from build123d import *

# Parameters (mm, degrees)
BOSS_EXTRUDE1_DEPTH = 10
SHELL1_START        = 1
SHELL1_DEPTH        = 9
CUT_EXTRUDE1_REACH  = 40.243
SKETCH2_W           = 4
SKETCH2_H           = 9


# Read off the part's stored shape, not the designer's step: Shell1
with BuildPart() as part:
    # Sketch1 → Boss-Extrude1 (new body)
    with BuildSketch(Plane.XY):
        with BuildLine():
            Line((-17.310520711, -21.823889376), (-3.597740248, -21.843555797))
            Line((-3.597740248, -21.843555797), (2.757908107, -14.842465178))
            ThreePointArc((2.757908107, -14.842465178), (-10.455115829, 18.525441507), (-23.668139764, -14.842465178))
            Line((-23.668139764, -14.842465178), (-17.310520711, -21.823889376))
        make_face()
    extrude(amount=BOSS_EXTRUDE1_DEPTH)

    # Shell1 outline → Shell1 (cut)
    with BuildSketch(Plane.XY.offset(SHELL1_START)):
        with BuildLine():
            Line((-4.039953619, -20.84292056), (2.044621953, -14.140431281))
            ThreePointArc((2.044621953, -14.140431281), (-10.45473176, 17.525441503), (-22.955414629, -14.139906596))
            Line((-22.955414629, -14.139906596), (-16.868083072, -20.824522877))
            Line((-16.868083072, -20.824522877), (-4.039953619, -20.84292056))
        make_face()
    extrude(amount=SHELL1_DEPTH, mode=Mode.SUBTRACT)

    # Sketch2 → Cut-Extrude1 (cut, up to next)
    with BuildSketch(Plane.XY.offset(10), mode=Mode.PRIVATE) as cut_extrude1_sk1:
        with Locations((-10.090473375, -2.029514736)):
            Rectangle(SKETCH2_W, SKETCH2_H)
    cut_extrude1_tool1 = extrude(cut_extrude1_sk1.sketch, amount=-CUT_EXTRUDE1_REACH, mode=Mode.PRIVATE) & part.part
    add(cut_extrude1_tool1.solids().sort_by_distance((-10.090473, -2.029515, 10))[0], mode=Mode.SUBTRACT)


solid = part.part
For this review, take the finished solid that the model builds, in its own axes (mm). A direction names the side the tool comes from. Round coordinates to 2 decimals unless told otherwise and drop trailing zeros. Loops run counter-clockwise (first coordinate to the right, second up) from the corner with the lowest first, then second, coordinate; pieces in that order, holes last. Notation, with made-up numbers: (-34, -8.75) - (-13, -8.75) arc R12 ccw to (-13, 3.25) - close; hole circle Ø1 at (-25.5, 52). An arc over 180 degrees is marked (long way). Use one line per item in the form item = value.
Item 1: Consider section D-D on y = -9.5. Write out the cut boundary in (x, z).
Answers:
outline = (-27.67, 0) - (6.76, 0) - (6.76, 10) - (5.63, 10) - (5.63, 1) - (-26.54, 1) - (-26.54, 10) - (-27.67, 10) - close
Item 2: Tool access review of faces 4 (the flat face through (5, -11, 10)), 5 (the flat face through (-7, -1, 1)), 6 (the flat face through (-12.09, -2.1, 0.5)): name each direction out of +Z, -Z, +X, -X, +Y, -Y from which nothing blocks a thin tool from reaching the whole face with its end or side.
Answers:
face_4 = +Z, +X, -X, +Y, -Y
face_5 = +Z
face_6 = +Z, -Z
Item 3: Clearance check with flat-ended pins moving along their axes: P1, Ø2, axis at x = -17, z = 5, coming from the -Y side; P2, Ø5, axis at x = -4.5, z = 4.5, coming from the +Y side; P3, Ø2, axis at x = -17, y = 6.5, coming from the +Z side. State where each tip first meets the part, or that it passes through.
Answers:
P1 = -21.83
P2 = 18.21
P3 = 1
Item 4: Consider section B-B on y = -4.5. Write out the cut boundary in (x, z).
Answers:
outline = (-29.39, 0) - (-12.09, 0) - (-12.09, 1) - (-28.37, 1) - (-28.37, 10) - (-29.39, 10) - close; (-8.09, 0) - (8.48, 0) - (8.48, 10) - (7.46, 10) - (7.46, 1) - (-8.09, 1) - close
Item 5: Consider section C-C on x = -15.5. Write out the cut boundary in (y, z).
Answers:
outline = (-21.83, 0) - (17.85, 0) - (17.85, 10) - (16.82, 10) - (16.82, 1) - (-20.83, 1) - (-20.83, 10) - (-21.83, 10) - close
Item 6: Consider section A-A on z = 3.25. Write out the cut boundary in (x, y), then the cut area to 3 significant figures.
Answers:
outline = (-23.67, -14.84) - (-17.31, -21.82) - (-3.6, -21.84) - (2.76, -14.84) arc R19.3 ccw (long way) to start; hole (-22.96, -14.14) - (-16.87, -20.82) - (-4.04, -20.84) - (2.04, -14.14) arc R18.3 ccw (long way) to start
area = 122 mm^2
Item 7: Mouldability with a two-part tool opening along Y and no side actions: class faces 1 (the flat face through (-6, -1, 0)), 2 (the cylindrical face through (-9.843, 17.515, 5.437)), 3 (the flat face through (-0.46, -18.39, 4.93)) as +Y half, -Y half, draft (parallel to the pull), parting line (faces both ways), or undercut.
Answers:
face_1 = draft
face_2 = undercut
face_3 = -Y half
Item 8: For line 1 (Y direction, x = -10, z = 3.75); line 2 (Z direction, x = 3, y = 0.5); line 3 (X direction, y = -5, z = 3.5), list the stretches that pass through material, from the lowest coordinate up.
Answers:
line_1 = -21.83 to -20.83, 17.52 to 18.52
line_2 = 0 to 1
line_3 = -29.29 to -28.26, 7.35 to 8.38
